CAD build for the part. Positions are in the model's coordinates, mm. Coordinates: 2 decimals unless noted, no trailing zeros. Loops run counter-clockwise (first coordinate to the right, second up) from the corner with the lowest first, then second, coordinate; pieces in that order, holes last. Notation, with made-up numbers: (85, -11.75) -> (134, -11.75) arc R21 cw to (134, 5.25) -> close; hole circle Ø6 at (82, 65). An arc over 180 degrees is marked (long way). Return JSON: item names as keys, results as strings. Group by question number.
(1) Probe L1, parallel to Y at x = -101, z = 13; L2, parallel to X at y = 219, z = 73.5; L3, parallel to Z at x = -112, y = 154. List the from-to ranges inside material, lowest first.
(2) Flat gauge pins, fed straight in: pin 1 Ø2 at (x, y) = (75, 137.5) entering from +Z; pin 2 Ø3 at (y, z) = (94.5, -87) entering from -X; pin 3 Ø3 at (y, z) = (213.5, -62.5) entering from -X. Where does each tip first touch, or does it go through?
(3) Saw through at B-B on z = 0. Write the cut outline in (x, y), then the cut area to 3 significant figures.
(4) Saw through at C-C on y = 54. Write the cut outline in (x, z).
(5) Saw through at A-A on x = 0. Write the cut outline in (y, z), then the cut area to 3 significant figures.
(6) Mould opens along Z. For faces 1 (the face through (-2, 0, 2)), 2 (the face through (-2, 1, -2)) say: pulls with the +Z half, pulls with the -Z half, needs draft (parallel to the pull), parting line crosses it, or undercut.
```python
from build123d import *


with BuildPart() as part:
    # ｽｹｯﾁ1 → 回転1 (revolve)
    with BuildSketch(Plane.XY, mode=Mode.PRIVATE) as revolve_1_sk:
        with BuildLine():
            Line((0, 0), (124.020829918, 0))
            Line((124.020829918, 0), (146.01902651, 251.440537606))
            ThreePointArc((146.01902651, 251.440537606), (151.218096937, 256), (156, 251.004758892))
            Line((156, 251.004758892), (157, 251.004758892))
            ThreePointArc((157, 251.004758892), (151.261716324, 256.999048222), (145.022831811, 251.527693349))
            Line((145.022831811, 251.527693349), (123.104498744, 1))
            Line((123.104498744, 1), (0, 1))
            Line((0, 1), (0, 0))
        make_face()
    revolve(revolve_1_sk.sketch.rotate(Axis((0, 1, 0), (0, -1, 0)), 90), axis=Axis((0, 1, 0), (0, -1, 0)))


solid = part.part
```
Geometry results:
{
 "1": {"L1": "0 to 1", "L2": "-122.88 to -121.7, 121.7 to 122.88", "L3": "-79.75 to -78.01, 78.01 to 79.75"},
 "2": {"pin 1": "z = 114.17", "pin 2": "x = -100.96", "pin 3": "x = -129.02"},
 "3": {"outline": "(-157, 251) -> (-156, 251) arc R5 cw to (-146.02, 251.44) -> (-124.02, 0) -> (124.02, 0) -> (146.02, 251.44) arc R5 cw to (156, 251) -> (157, 251) arc R6 ccw to (145.02, 251.53) -> (123.1, 1) -> (-123.1, 1) -> (-145.02, 251.53) arc R6 ccw to start", "area": "785 mm²"},
 "4": {"outline": "circle Ø257.49 at (0, 0); hole circle Ø255.48 at (0, 0)"},
 "5": {"outline": "(0, -124.02) -> (251.44, -146.02) arc R5 cw to (251, -156) -> (251, -157) arc R6 ccw to (251.53, -145.02) -> (1, -123.1) -> (1, 123.1) -> (251.53, 145.02) arc R6 ccw to (251, 157) -> (251, 156) arc R5 cw to (251.44, 146.02) -> (0, 124.02) -> close", "area": "785 mm²"},
 "6": {"face 1": "needs draft", "face 2": "undercut"}
}
